Work out the finished part from the listing and answer in its coordinate system (mm). Face numbers are marked on the shaded views. A direction names the side the tool comes from. Round coordinates to 2 decimals unless told otherwise and drop trailing zeros. Loops run counter-clockwise (first coordinate to the right, second up) from the corner with the lowest first, then second, coordinate; pieces in that order, holes last. Notation, with made-up numbers: (30.25, 0.5) - (51.25, 0.5) arc R14 ccw to (51.25, 25.5) - close; hole circle Ø9 at (-11, 58.5). An arc over 180 degrees is marked (long way). Return JSON: item names as keys, results as strings.
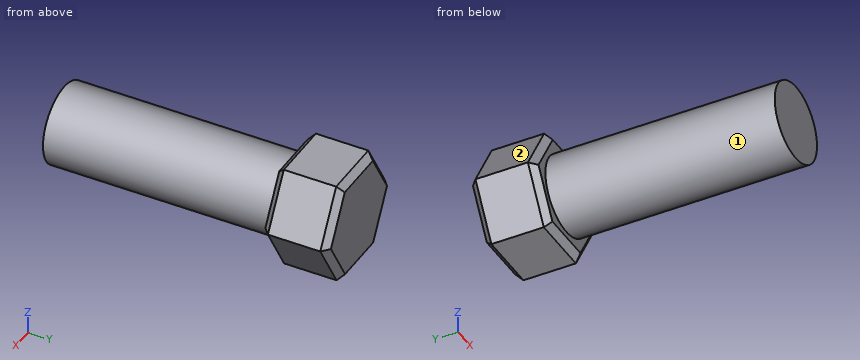
from build123d import *

# Parameters (mm, degrees)
CROQUIS2_R              = 6
SALIENTE_EXTRUIR1_DEPTH = 35
SALIENTE_EXTRUIR2_DEPTH = 10
CHAFL_N1_SIZE           = 1


with BuildPart() as part:
    # Croquis2 → Saliente-Extruir1 (new body)
    with BuildSketch(Plane(origin=(0, 0, 0), x_dir=(1, 0, 0), z_dir=(0, 1, 0))):
        with Locations(Location((0, 0, 0), (0, 0, 270))):
            Circle(CROQUIS2_R)
    extrude(amount=SALIENTE_EXTRUIR1_DEPTH)

    # Croquis3 → Saliente-Extruir2 (add)
    with BuildSketch(Plane(origin=(0, 35, 0), x_dir=(1, 0, 0), z_dir=(0, 1, 0))):
        Polygon((4.607833062, -7.866269978), (9.116306165, 0.057365499), (4.508473103, 7.923635477), (-4.607833062, 7.866269978), (-9.116306165, -0.057365499), (-4.508473103, -7.923635477), align=None)
    extrude(amount=SALIENTE_EXTRUIR2_DEPTH)

    # Chaflán1
    chafl_n1_edges = [part.edges().sort_by_distance(p)[0] for p in [
        (0.04967998, 35, 7.894952727),
        (6.862069613, 35, 3.904452239),
        (6.812389634, 35, -3.990500488),
        (-0.04967998, 35, -7.894952727),
        (-6.862069613, 35, -3.904452239),
        (-6.812389634, 35, 3.990500488),
        (0.04967998, 45, 7.894952727),
        (6.862069613, 45, 3.904452239),
        (6.812389634, 45, -3.990500488),
        (-0.04967998, 45, -7.894952727),
        (-6.862069613, 45, -3.904452239),
        (-6.812389634, 45, 3.990500488),
    ]]
    chamfer(chafl_n1_edges, length=CHAFL_N1_SIZE)


solid = part.part
1) Section B-B (y = 38.5) is taken. Give the vertices of the cut face in (x, z), and give its area (3 significant figures).
Verdict:
{"outline": "(-9.12, 0.06) - (-4.61, -7.87) - (4.51, -7.92) - (9.12, -0.06) - (4.61, 7.87) - (-4.51, 7.92) - close", "area": "216 mm2"}
2) Flat-ended cylindrical pins translate along their axes: pin 1 (5 mm diameter, centred on x = -3.5, y = 29, fed in from +Z); pin 2 (4 mm diameter, centred on x = -3.5, z = 3, fed in from -Y); pin 3 (5 mm diameter, centred on y = 14, z = -3, fed in from -X); pin 4 (5 mm diameter, centred on x = 6, y = 20, fed in from +Z). Find the tip coordinate at first contact, or state that the pin passes through.
Verdict:
{"pin 1": "stops at z = 5.92", "pin 2": "stops at y = 0", "pin 3": "stops at x = -5.98", "pin 4": "stops at z = 4.87"}
3) A tool of negligible diameter and unlimited length cuts with its end or side. For the marked faces 1 and 2, from which of +Z, -Z, +X, -X, +Y, -Y can it reach the whole face along a straight path? Write none if from no direction.
Verdict:
{"face 1": "-Y", "face 2": "+Z, -X, +Y, -Y"}
4) Section A-A (z = -2.25) is taken. Give the vertices of the cut face in (x, y), and give its area (3 significant figures).
Verdict:
{"outline": "(-7.8, 36) - (-6.65, 35) - (-5.56, 35) - (-5.56, 0) - (5.56, 0) - (5.56, 35) - (6.67, 35) - (7.83, 36) - (7.83, 44) - (6.67, 45) - (-6.65, 45) - (-7.8, 44) - close", "area": "543 mm2"}
5) Section C-C (x = 0) is taken. Give the vertices of the cut face in (y, z), and give its area (3 significant figures).
Verdict:
{"outline": "(0, -6) - (35, -6) - (35, -6.9) - (36, -7.9) - (44, -7.9) - (45, -6.9) - (45, 6.9) - (44, 7.9) - (36, 7.9) - (35, 6.9) - (35, 6) - (0, 6) - close", "area": "576 mm2"}
6) Find the intervals of material crossed by L1, parallel to Y at x = 0, z = 6.5; L2, parallel to Z at x = 4.5, y = 39; L3, parallel to Z at x = 1.75, y = 17.5, in increasing order.
Verdict:
{"L1": "y = 35 to 45", "L2": "z = -7.92 to 7.87", "L3": "z = -5.74 to 5.74"}
7) Section D-D (y = 8.5) is taken. Give the vertices of the cut face in (x, z).
Verdict:
{"outline": "circle Ø12 at (0, 0)"}
